Design review of the part built by this model. Coordinates are the model's own, in mm. Face numbers are marked on the shaded views. A direction names the side the tool comes from. Coordinates: 2 decimals unless noted, no trailing zeros. Write each loop counter-clockwise with the first axis right and the second up, starting at its lowest first coordinate (ties: lowest second). Pieces come first, ordered by that corner, then holes.
Q1. Machinability: for the marked faces 1 and 2, which of the approach directions +Z, -Z, +X, -X, +Y, -Y give a long, thin tool a straight path to every point of the face, cutting with its end or side? Answer none if there is none.
Q2. Take a section at B-B (x = 30). Give the boundary of the cut face in (y, z).
Q3. For probe 1 along Y at (x, z) = (50, 0.65); probe 2 along Z at (x, y) = (28.5, 28.5); probe 3 along Y at (x, z) = (55, 1.9), list the stretches that pass through material, from the lowest coordinate up.
Q4. Take a section at A-A (y = 20). Give the boundary of the cut face in (x, z), and give its area (3 significant figures).
Q5. Take a section at C-C (x = 55). Give the boundary of the cut face in (y, z).
Q6. Insertion check: pin 1 (5 mm diameter, centred on x = 18, z = 4, fed in from +Y); pin 2 (2 mm diameter, centred on x = 50.5, z = 10, fed in from +Y); pin 3 (22.5 mm diameter, centred on x = 23, y = 29.5, fed in from +Z). Each pin has a flat end and moves straight along its axis. Give the tip position at first contact, or say it passes through.
Q7. Take a section at D-D (y = 10). Give the boundary of the cut face in (x, z).
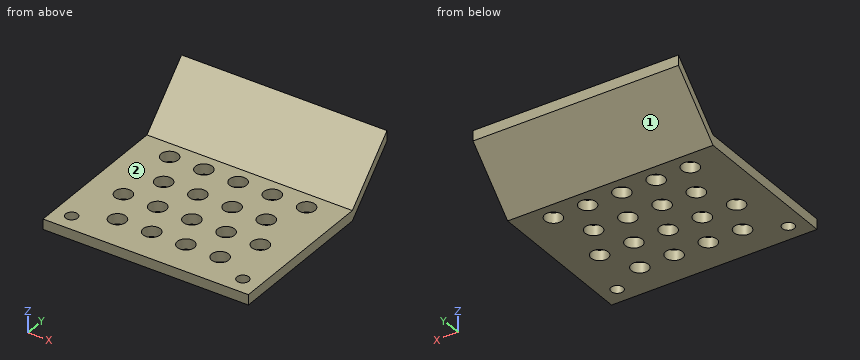
Autodesk Inventor part; units mm, degrees
ref_plane "YZ Plane" through (0, 0, 0) normal (1, 0, 0) x (0, 1, 0)
ref_plane "XZ Plane" through (0, 0, 0) normal (0, 1, 0) x (-1, 0, 0)
ref_plane "XY Plane" through (0, 0, 0) normal (0, 0, 1) x (1, 0, 0)
sketch "Sketch3" plane through (0, 0, 0) normal (1, 0, 0) x (0, 1, 0)
  line L0 (0, 0) -> (45, 0)
  line L1 (45, 0) -> (60, 15)
  line L2 (0, 0) -> (0, 3)
  line L3 (0, 3) -> (45, 3)
  line L4 (45, 3) -> (60, 18)
  line L5 (60, 18) -> (60, 15)
  dimension "d7" = 45
  dimension "d8" = 135
  dimension "d10" = 15
  dimension "d11" = 45
  dimension "d12" = 21.2132
  dimension "d13" = 3
extrude "Extrusion3" add sketch "Sketch3" along normal blind 60
sketch "Sketch4" plane through (0, 0, 0) normal (0, 0, -1) x (-1, 0, 0)
  line L0 (0, 0) -> (0, 45)
  line L1 (0, 45) -> (-60, 45)
  line L2 (-60, 0) -> (-60, 45)
  line L3 (0, 0) -> (-60, 0)
  circle A0 centre (-55, 5) radius 1.75
  circle A1 centre (-5, 5) radius 1.75
  dimension "d16" = 3.5
  dimension "d18" = 50
  dimension "d19" = 5
extrude "Extrusion4" cut sketch "Sketch4" against normal through all contours A0 | A1
sketch "Sketch5" plane through (0, 0, 3) normal (0, 0, 1) x (1, 0, 0)
  circle A0 centre (55, 5) radius 1.75
  circle A1 centre (5, 5) radius 1.75
  line L0 (0, 45) -> (0, 0)
  line L1 (0, 0) -> (60, 0)
  line L2 (60, 45) -> (60, 0)
  line L3 (0, 45) -> (60, 45)
  circle A2 centre (10, 40) radius 2.5
  circle A3 centre (20, 40) radius 2.5
  circle A4 centre (30, 40) radius 2.5
  circle A5 centre (40, 40) radius 2.5
  circle A6 centre (50, 40) radius 2.5
  circle A7 centre (10, 20) radius 2.5
  circle A8 centre (20, 20) radius 2.5
  circle A9 centre (30, 20) radius 2.5
  circle A10 centre (40, 20) radius 2.5
  circle A11 centre (50, 20) radius 2.5
  circle A12 centre (15, 30) radius 2.5
  circle A13 centre (25, 30) radius 2.5
  circle A14 centre (35, 30) radius 2.5
  circle A15 centre (45, 30) radius 2.5
  circle A16 centre (15, 10) radius 2.5
  circle A17 centre (25, 10) radius 2.5
  circle A18 centre (35, 10) radius 2.5
  circle A19 centre (45, 10) radius 2.5
  point P0 (0, 0)
  dimension "d22" = 5
  dimension "d25" = 10
  dimension "d28" = 20
  dimension "d32" = 5
  dimension "d33" = 10
  dimension "d35" = 10
  dimension "d38" = 10
  dimension "d41" = 20
extrude "Extrusion5" cut sketch "Sketch5" against normal through all contours A2 | A3 | A4 | A5 | A6 | A7 | A8 | A9 | A10 | A11 | A12 | A13 | A14 | A15 | A16 | A17 | A18 | A19
properties part number "rejilla.ventilador"
Response:
1. face 1: -Z, +X, -X, +Y
1. face 2: +Z, +X, -X, -Y
2. outline: (0, 0) - (17.5, 0) - (17.5, 3) - (0, 3) - close; (22.5, 0) - (37.5, 0) - (37.5, 3) - (22.5, 3) - close; (42.5, 0) - (45, 0) - (60, 15) - (60, 18) - (45, 3) - (42.5, 3) - close
3. probe 1: y = 0 to 17.5, 22.5 to 37.5, 42.5 to 45.65
3. probe 2: z = 0 to 3
3. probe 3: y = 0 to 3.25, 6.75 to 46.9
4. outline: (0, 0) - (7.5, 0) - (7.5, 3) - (0, 3) - close; (12.5, 0) - (17.5, 0) - (17.5, 3) - (12.5, 3) - close; (22.5, 0) - (27.5, 0) - (27.5, 3) - (22.5, 3) - close; (32.5, 0) - (37.5, 0) - (37.5, 3) - (32.5, 3) - close; (42.5, 0) - (47.5, 0) - (47.5, 3) - (42.5, 3) - close; (52.5, 0) - (60, 0) - (60, 3) - (52.5, 3) - close
4. area: 105 mm2
5. outline: (0, 0) - (3.25, 0) - (3.25, 3) - (0, 3) - close; (6.75, 0) - (45, 0) - (60, 15) - (60, 18) - (45, 3) - (6.75, 3) - close
6. pin 1: stops at y = 51.5
6. pin 2: stops at y = 56
6. pin 3: stops at z = 3
7. outline: (0, 0) - (12.5, 0) - (12.5, 3) - (0, 3) - close; (17.5, 0) - (22.5, 0) - (22.5, 3) - (17.5, 3) - close; (27.5, 0) - (32.5, 0) - (32.5, 3) - (27.5, 3) - close; (37.5, 0) - (42.5, 0) - (42.5, 3) - (37.5, 3) - close; (47.5, 0) - (60, 0) - (60, 3) - (47.5, 3) - close
